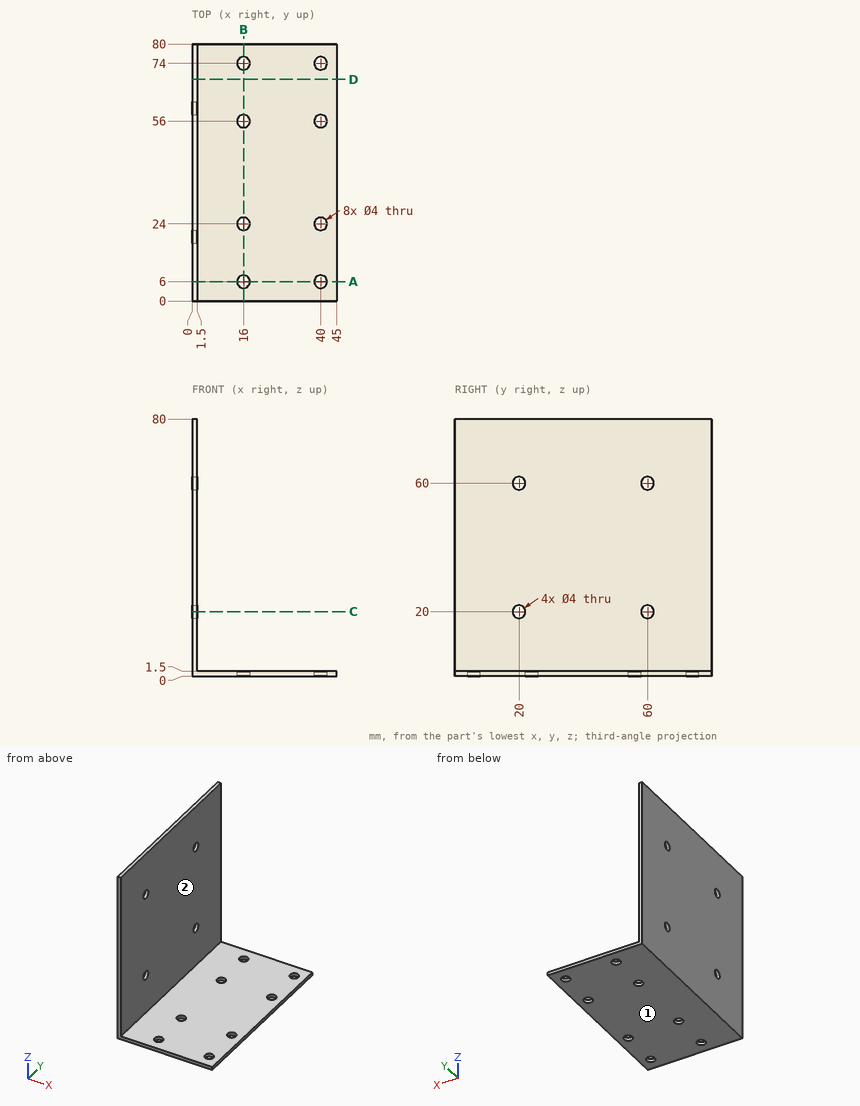
For this review, use the dimensioned drawing (mm, ordinates from the lowest corner) and the shaded views. A direction names the side the tool comes from. Coordinates: 2 decimals unless noted, no trailing zeros. Loops run counter-clockwise (first coordinate to the right, second up) from the corner with the lowest first, then second, coordinate; pieces in that order, holes last.
1. Add section B-B, the plane x = 16. Give the boundary of the cut face in (y, z).
2. Add section C-C, the plane z = 20. Give the boundary of the cut face in (x, y), then the cut area to 3 significant figures.
3. Insertion check: P1, Ø3, axis at y = 20, z = 60, coming from the -X side; P2, Ø1.5, axis at y = 35, z = 20, coming from the +X side; P3, Ø6.5, axis at x = 40, y = 74, coming from the +Z side. Each pin has a flat end and moves straight along its axis. Give the tip position at first contact, or say it passes through.
4. For line 1 (Y direction, x = 16, z = 0.5); line 2 (Z direction, x = 0.3, y = 20); line 3 (X direction, y = 24, z = 0.6), list the stretches that pass through material, from the lowest coordinate up.
5. Add section D-D, the plane y = 69. Give the boundary of the cut face in (x, z), then the cut area to 3 significant figures.
6. For the marked faces 1 and 2, list the 3-axis set-ups (+Z, -Z, +X, -X, +Y, -Y) from which the entire face can be reached by the end or side of a thin tool; tool diameter is ignored.
7. Add section A-A, the plane y = 6. Give the boundary of the cut face in (x, z), then the cut area to 3 significant figures.
Result:
1. outline: (0, 0) - (4, 0) - (4, 1.5) - (0, 1.5) - close; (8, 0) - (22, 0) - (22, 1.5) - (8, 1.5) - close; (26, 0) - (54, 0) - (54, 1.5) - (26, 1.5) - close; (58, 0) - (72, 0) - (72, 1.5) - (58, 1.5) - close; (76, 0) - (80, 0) - (80, 1.5) - (76, 1.5) - close
2. outline: (0, 0) - (1.5, 0) - (1.5, 18) - (0, 18) - close; (0, 22) - (1.5, 22) - (1.5, 58) - (0, 58) - close; (0, 62) - (1.5, 62) - (1.5, 80) - (0, 80) - close
2. area: 108 mm2
3. P1: passes through
3. P2: stops at x = 1.5
3. P3: stops at z = 1.5
4. line 1: y = 0 to 4, 8 to 22, 26 to 54, 58 to 72, 76 to 80
4. line 2: z = 0 to 18, 22 to 58, 62 to 80
4. line 3: x = 0 to 14, 18 to 38, 42 to 45
5. outline: (0, 0) - (45, 0) - (45, 1.5) - (1.5, 1.5) - (1.5, 80) - (0, 80) - close
5. area: 185 mm2
6. face 1: -Z, +X, -X, +Y, -Y
6. face 2: +Z, +X, +Y, -Y
7. outline: (0, 0) - (14, 0) - (14, 1.5) - (1.5, 1.5) - (1.5, 80) - (0, 80) - close; (18, 0) - (38, 0) - (38, 1.5) - (18, 1.5) - close; (42, 0) - (45, 0) - (45, 1.5) - (42, 1.5) - close
7. area: 173 mm2
